from build123d import *

# Parameters (mm, degrees)
F0_W     = 101.6
F0_H     = 101.6
F1_DEPTH = 25.4
F3_DEPTH = 101.6
F4_W     = 101.6
F4_H     = 101.6
F5_DEPTH = 25.4
F6_DEPTH = 25.4


with BuildPart() as f1:
    # F0 (on Top) → F1 (new body)
    with BuildSketch(Plane.XY):
        with Locations((50.8, -50.8)):
            Rectangle(F0_W, F0_H)
    extrude(amount=F1_DEPTH)

    # F2 (on face) → F3 (join)
    with BuildSketch(Plane.XY.offset(25.4)):
        Polygon((101.6, 0), (0, 0), (101.6, -101.6), align=None)
    extrude(amount=F3_DEPTH)

    # F4 (on face) → F5 (join)
    with BuildSketch(Plane.XY.offset(127)):
        with Locations((50.8, -50.8)):
            Rectangle(F4_W, F4_H)
    extrude(amount=F5_DEPTH)

    # F5_face (on face) → F6 (join)
    with BuildSketch(Plane(origin=(101.6, -50.8, 76.2), x_dir=(0, 1, 0), z_dir=(1, 0, 0))):
        Polygon((-50.8, -50.8), (-50.8, -76.2), (50.8, -76.2), (50.8, 76.2), (-50.8, 76.2), (-50.8, 50.8), align=None)
    extrude(amount=F6_DEPTH)


solid = f1.part
Design review of the part built by this model. Coordinates are the model's own, in mm. A direction names the side the tool comes from. Coordinates: 2 decimals unless noted, no trailing zeros. Order: outer loops, then holes, each group sorted by start corner. A loop starts at its lowest first (then second) coordinate and runs counter-clockwise, first axis right, second up.
Item 1: Take a section at B-B, the plane x = 85. Write out the cut boundary in (y, z).
Item 2: Take a section at C-C, the plane z = 101.5. Write out the cut boundary in (x, y).
Item 3: For line 1 (Z direction, x = 41, y = -60); line 2 (X direction, y = -87.5, z = 75.5); line 3 (Y direction, x = 38, z = 99.5), list the stretches that pass through material, from the lowest coordinate up.
Item 4: Take a section at A-A, the plane y = -41. Write out the cut boundary in (x, z), then the cut area to 3 significant figures.
Item 5: For faces 4 (the flat face through (28, -73, 25.4)), 5 (the flat face through (127, -52, 77)), list the 3-axis set-ups (+Z, -Z, +X, -X, +Y, -Y) from which the entire face can be reached by the end or side of a thin tool; tool diameter is ignored.
Item 6: For pin 1 Ø1 at (x, z) = (91, 122.5) entering from -Y; pin 2 Ø5 at (x, z) = (46.5, 98) entering from -Y; pin 3 Ø10 at (x, z) = (14, 42.5) entering from -Y, all flat-tipped, find the tip position at first contact; note any pin that passes through.
Item 7: The part is to be moulded in two halves that separate along Z. For faces 1 (the flat face through (0, -52, 13)), 2 (the flat face through (63, -52, 0)), 3 (the flat face through (50, -50, 75)), say which applies: pulls with the +Z half, pulls with the -Z half, needs draft (parallel to the pull), parting line crosses it, or undercut.
The answers:
1. outline: (-101.6, 0) - (0, 0) - (0, 152.4) - (-101.6, 152.4) - (-101.6, 127) - (-85, 127) - (-85, 25.4) - (-101.6, 25.4) - close
2. outline: (0, 0) - (101.6, -101.6) - (127, -101.6) - (127, 0) - close
3. line 1: z = 0 to 25.4, 127 to 152.4
3. line 2: x = 87.5 to 127
3. line 3: y = -38 to 0
4. outline: (0, 0) - (127, 0) - (127, 152.4) - (0, 152.4) - (0, 127) - (41, 127) - (41, 25.4) - (0, 25.4) - close
4. area: 15,200 mm2
5. face 4: -X, -Y
5. face 5: +Z, -Z, +X, +Y, -Y
6. pin 1: stops at y = -91.5
6. pin 2: stops at y = -49
6. pin 3: stops at y = -19
7. face 1: needs draft
7. face 2: pulls with the -Z half
7. face 3: undercut
